Geometry check sheet. Reference: the model listing, model coordinates, mm. Face numbers are marked on the shaded views. Round coordinates to 2 decimals unless told otherwise and drop trailing zeros. Order: outer loops, then holes, each group sorted by start corner. A loop starts at its lowest first (then second) coordinate and runs counter-clockwise, first axis right, second up. Notation, with made-up numbers: (8.25, 38) -> (15.25, 38) arc R13 cw to (15.25, 54) -> close; hole circle Ø2 at (9.5, -38.75). An arc over 180 degrees is marked (long way). Use a Markdown table: item, result. Add a question column.
Item 1: Material ranges on probe 1 along Y at (x, z) = (21.5, 3.5); probe 2 along X at (y, z) = (13.5, 5); probe 3 along Y at (x, z) = (33, 4.5), recorded low to high. Write a range as [from, to].
Item 2: Mould release check, pull along X, two halves, no side actions. Record for the marked faces 1 and 2: pulls with the +X half, pulls with the -X half, needs draft (parallel to the pull), parting line crosses it, or undercut.
Item 3: Sectioned sample at B-B, the plane x = 58.5. Record the cut outline in (y, z), and give its area (3 significant figures).
Item 4: Sectioned sample at C-C, the plane y = 28. Record the cut outline in (x, z), and give its area (3 significant figures).
Item 5: Sectioned sample at A-A, the plane z = 5. Record the cut outline in (x, y).
Item 6: Gauge pin test, flat ends, axial feed: pin 1 Ø1 at (y, z) = (31, 5.5) entering from -X; pin 2 Ø2.5 at (x, z) = (70.5, 5.5) entering from -Y; pin 3 Ø3 at (x, y) = (22, 42.5) entering from +Z. Record the tip position at first contact, or that the pin passes through.
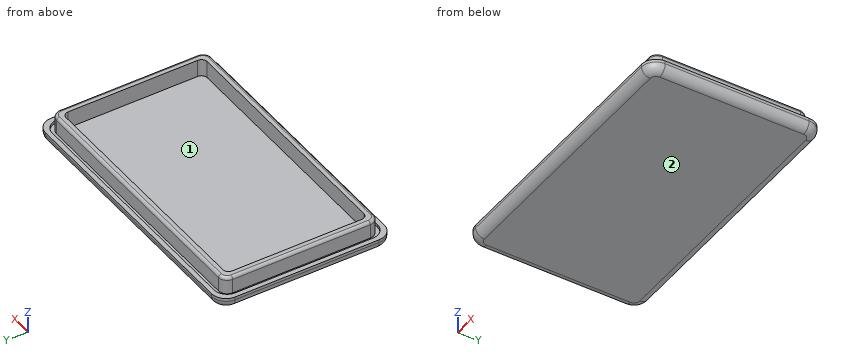
from build123d import *

# Parameters (mm, degrees)
SKETCH_W        = 100
SKETCH_H        = 60
PAD_DEPTH       = 4
FILLET_R        = 5
FILLET001_R     = 3
POCKET001_DEPTH = 1
PAD001_DEPTH    = 5
POCKET_DEPTH    = 6
FILLET002_R     = 1


with BuildPart() as part:
    # Sketch → Pad (new body)
    with BuildSketch(Plane.XY):
        with Locations((50, 30)):
            Rectangle(SKETCH_W, SKETCH_H)
    extrude(amount=PAD_DEPTH)

    # Fillet
    fillet_edges = [part.edges().sort_by_distance(p)[0] for p in [
        (100, 0, 2),
        (0, 0, 2),
        (100, 60, 2),
        (0, 60, 2),
    ]]
    fillet(fillet_edges, radius=FILLET_R)

    # Fillet001
    fillet001_edges = [part.edges().sort_by_distance(p)[0] for p in [
        (50, 60, 0),
    ]]
    fillet(fillet001_edges, radius=FILLET001_R)

    # Sketch008 (on Face6 of Pad) → Pocket001 (cut)
    with BuildSketch(Plane.XY.offset(4)):
        with BuildLine():
            Line((6.1, 1.6), (93.9, 1.6))
            ThreePointArc((93.9, 1.6), (97.081981, 2.918019), (98.4, 6.1))
            Line((98.4, 6.1), (98.4, 53.9))
            ThreePointArc((98.4, 53.9), (97.081981, 57.081981), (93.9, 58.4))
            Line((93.9, 58.4), (6.1, 58.4))
            ThreePointArc((6.1, 58.4), (2.918019, 57.081981), (1.6, 53.9))
            Line((1.6, 53.9), (1.6, 6.1))
            ThreePointArc((1.6, 6.1), (2.918019, 2.918019), (6.1, 1.6))
        make_face()
        with BuildLine():
            Line((6.1, 3.1), (93.9, 3.1))
            ThreePointArc((93.9, 3.1), (96.02132, 3.97868), (96.9, 6.1))
            Line((96.9, 6.1), (96.9, 53.9))
            ThreePointArc((96.9, 53.9), (96.02132, 56.02132), (93.9, 56.9))
            Line((93.9, 56.9), (6.1, 56.9))
            ThreePointArc((6.1, 56.9), (3.97868, 56.02132), (3.1, 53.9))
            Line((3.1, 53.9), (3.1, 6.1))
            ThreePointArc((3.1, 6.1), (3.97868, 3.97868), (6.1, 3.1))
        make_face(mode=Mode.SUBTRACT)
    extrude(amount=-POCKET001_DEPTH, mode=Mode.SUBTRACT)

    # Sketch001 (on Face6 of Pad) → Pad001 (join)
    with BuildSketch(Plane.XY.offset(4)):
        with BuildLine():
            Line((6.1, 3.1), (93.9, 3.1))
            ThreePointArc((93.9, 3.1), (96.02132, 3.97868), (96.9, 6.1))
            Line((96.9, 6.1), (96.9, 53.9))
            ThreePointArc((96.9, 53.9), (96.02132, 56.02132), (93.9, 56.9))
            Line((93.9, 56.9), (6.1, 56.9))
            ThreePointArc((6.1, 56.9), (3.97868, 56.02132), (3.1, 53.9))
            Line((3.1, 53.9), (3.1, 6.1))
            ThreePointArc((3.1, 6.1), (3.97868, 3.97868), (6.1, 3.1))
        make_face()
    extrude(amount=PAD001_DEPTH)

    # Sketch009 (on Face44 of Pad001) → Pocket (cut)
    with BuildSketch(Plane.XY.offset(9)):
        with BuildLine():
            Line((7.5, 5.5), (92.5, 5.5))
            ThreePointArc((92.5, 5.5), (93.914214, 6.085786), (94.5, 7.5))
            Line((94.5, 7.5), (94.5, 52.5))
            ThreePointArc((94.5, 52.5), (93.914214, 53.914214), (92.5, 54.5))
            Line((92.5, 54.5), (7.5, 54.5))
            ThreePointArc((7.5, 54.5), (6.085786, 53.914214), (5.5, 52.5))
            Line((5.5, 52.5), (5.5, 7.5))
            ThreePointArc((5.5, 7.5), (6.085786, 6.085786), (7.5, 5.5))
        make_face()
    extrude(amount=-POCKET_DEPTH, mode=Mode.SUBTRACT)

    # Fillet002
    fillet002_edges = [part.edges().sort_by_distance(p)[0] for p in [
        (50, 3.1, 9),
    ]]
    fillet(fillet002_edges, radius=FILLET002_R)


solid = part.part
Found:
| question | item | result |
|---|---|---|
| 1 | probe 1 | y = [0, 1.6], [3.1, 5.5], [54.5, 56.9], [58.4, 60] |
| 1 | probe 2 | x = [3.1, 5.5], [94.5, 96.9] |
| 1 | probe 3 | y = [3.1, 5.5], [54.5, 56.9] |
| 2 | face 1 | undercut |
| 2 | face 2 | needs draft |
| 3 | outline | (0, 3) arc R3 ccw to (3, 0) -> (57, 0) arc R3 ccw to (60, 3) -> (60, 4) -> (58.4, 4) -> (58.4, 3) -> (56.9, 3) -> (56.9, 8) arc R1 ccw to (55.9, 9) -> (54.5, 9) -> (54.5, 3) -> (5.5, 3) -> (5.5, 9) -> (4.1, 9) arc R1 ccw to (3.1, 8) -> (3.1, 3) -> (1.6, 3) -> (1.6, 4) -> (0, 4) -> close |
| 3 | area | 208 mm2 |
| 4 | outline | (0, 3) arc R3 ccw to (3, 0) -> (97, 0) arc R3 ccw to (100, 3) -> (100, 4) -> (98.4, 4) -> (98.4, 3) -> (96.9, 3) -> (96.9, 8) arc R1 ccw to (95.9, 9) -> (94.5, 9) -> (94.5, 3) -> (5.5, 3) -> (5.5, 9) -> (4.1, 9) arc R1 ccw to (3.1, 8) -> (3.1, 3) -> (1.6, 3) -> (1.6, 4) -> (0, 4) -> close |
| 4 | area | 328 mm2 |
| 5 | outline | (3.1, 6.1) arc R3 ccw to (6.1, 3.1) -> (93.9, 3.1) arc R3 ccw to (96.9, 6.1) -> (96.9, 53.9) arc R3 ccw to (93.9, 56.9) -> (6.1, 56.9) arc R3 ccw to (3.1, 53.9) -> close; hole (5.5, 7.5) arc R2 ccw to (7.5, 5.5) -> (92.5, 5.5) arc R2 ccw to (94.5, 7.5) -> (94.5, 52.5) arc R2 ccw to (92.5, 54.5) -> (7.5, 54.5) arc R2 ccw to (5.5, 52.5) -> close |
| 6 | pin 1 | stops at x = 3.1 |
| 6 | pin 2 | stops at y = 3.1 |
| 6 | pin 3 | stops at z = 3 |
